from build123d import *

# Parameters (mm, degrees)
EXTRUDE1_DEPTH = 6.35
FILLET1_R      = 6.35


with BuildPart() as part:
    # Sketch1 → Extrude1 (new body)
    with BuildSketch(Plane.XY):
        with BuildLine():
            Line((-101.6, 0), (-76.2, 0))
            ThreePointArc((-76.2, 0), (-68.760512242, -17.960512242), (-50.8, -25.4))
            Line((-50.8, -25.4), (50.8, -25.4))
            ThreePointArc((50.8, -25.4), (68.760512242, -17.960512242), (76.2, 0))
            Line((76.2, 0), (101.6, 0))
            Line((101.6, 0), (101.6, -63.5))
            Line((101.6, -63.5), (-101.6, -63.5))
            Line((-101.6, -63.5), (-101.6, 0))
        make_face()
    extrude(amount=EXTRUDE1_DEPTH)

    # Fillet1
    fillet1_edges = [part.edges().sort_by_distance(p)[0] for p in [
        (101.6, -63.5, 3.175),
        (-101.6, -63.5, 3.175),
    ]]
    fillet(fillet1_edges, radius=FILLET1_R)


solid = part.part
Read the model definition and answer for the solid it produces. Units are mm, in the model's axes. A direction names the side the tool comes from. Coordinates: 2 decimals unless noted, no trailing zeros. Write each loop counter-clockwise with the first axis right and the second up, starting at its lowest first coordinate (ties: lowest second). Pieces come first, ordered by that corner, then holes. Notation, with made-up numbers: (84.5, -38) -> (93.5, -38) arc R22 cw to (93.5, -24) -> close; hole circle Ø9 at (4, 58). An arc over 180 degrees is marked (long way). Return JSON: item names as keys, results as strings.
(1) Which of the six approach directions +Z, -Z, +X, -X, +Y, -Y give full straight-line access (tool end or side, diameter ignored) to faces 5 (the cylindrical face through (-99.69, -61.69, 3.22)), 6 (the cylindrical face through (-68.96, -17.76, 3.13))?
Answers below:
{"face 5": "+Z, -Z, -X, -Y", "face 6": "+Z, -Z, +Y"}
(2) The part is cut by section C-C on x = 3. Give the vertices of the cut face in (y, z).
Answers below:
{"outline": "(-63.5, 0) -> (-25.4, 0) -> (-25.4, 6.35) -> (-63.5, 6.35) -> close"}
(3) For a pull along X with two mould halves and no side action, classify faces 1 (the flat face through (89, 0, 3)), 2 (the cylindrical face through (68.56, -18.16, 3.13)), 3 (the flat face through (-1, -25.4, 3)), 4 (the flat face through (-101.6, -29, 3)) as pulls with the +X half, pulls with the -X half, needs draft (parallel to the pull), parting line crosses it, or undercut.
Answers below:
{"face 1": "needs draft", "face 2": "undercut", "face 3": "undercut", "face 4": "pulls with the -X half"}
(4) The part is cut by section B-B on y = -14. Give the vertices of the cut face in (x, z).
Answers below:
{"outline": "(-101.6, 0) -> (-71.99, 0) -> (-71.99, 6.35) -> (-101.6, 6.35) -> close; (71.99, 0) -> (101.6, 0) -> (101.6, 6.35) -> (71.99, 6.35) -> close"}
(5) The part is cut by section A-A on z = 1.5. Give the vertices of the cut face in (x, y).
Answers below:
{"outline": "(-101.6, -57.15) arc R6.35 ccw to (-95.25, -63.5) -> (95.25, -63.5) arc R6.35 ccw to (101.6, -57.15) -> (101.6, 0) -> (76.2, 0) arc R25.4 cw to (50.8, -25.4) -> (-50.8, -25.4) arc R25.4 cw to (-76.2, 0) -> (-101.6, 0) -> close"}
(6) Each of these flat-tipped pins is pushed along its axis until it touches: P1, Ø1.9, axis at x = 7, z = 2, coming from the +Y side; P2, Ø3, axis at x = 69.5, z = 4.5, coming from the +Y side. Where does it stop, or does it pass through?
Answers below:
{"P1": "y = -25.4", "P2": "y = -15.4"}
(7) The part is cut by section D-D on x = -70.5. Give the vertices of the cut face in (y, z).
Answers below:
{"outline": "(-63.5, 0) -> (-16.03, 0) -> (-16.03, 6.35) -> (-63.5, 6.35) -> close"}
(8) Consider line 1 along X through (y, z) = (-22.5, 2.75); line 2 along X through (y, z) = (-6.5, 3.5); line 3 along Y through (x, z) = (-39, 2.5). Determine where each line is inside the solid, lowest interval first. Write a range as from..to.
Answers below:
{"line 1": "-101.6..-62.59, 62.59..101.6", "line 2": "-101.6..-75.35, 75.35..101.6", "line 3": "-63.5..-25.4"}
